CAD build for the part. Positions are in the model's coordinates, mm. Face numbers are marked on the shaded views. A direction names the side the tool comes from. Round coordinates to 2 decimals unless told otherwise and drop trailing zeros. Loops run counter-clockwise (first coordinate to the right, second up) from the corner with the lowest first, then second, coordinate; pieces in that order, holes last. Notation, with made-up numbers: M 40,61.25 L 89,61.25 A18 cw 89,94.25 Z; hole C 12,33 d8. An arc over 180 degrees is marked long. Use one line per item in the form item = value.
from build123d import *

# Parameters (mm, degrees)
F0_R     = 7.9375
F1_DEPTH = 3.175
F2_R     = 5.55625
F3_DEPTH = 11.1125
F5_DEPTH = 6.35
F6_SIZE  = 0.508


with BuildPart() as f1:
    # F0 (on Top) → F1 (new body)
    with BuildSketch(Plane.XY):
        Circle(F0_R)
    extrude(amount=F1_DEPTH)

    # F2 (on face) → F3 (join)
    with BuildSketch(Plane.XY.offset(3.175)):
        Circle(F2_R)
    extrude(amount=F3_DEPTH)

    # F4 (on face) → F5 (cut)
    with BuildSketch(Plane(origin=(0, 0, 0), x_dir=(1, 0, 0), z_dir=(0, 0, -1))):
        Polygon((-3.056609, -1.764734), (0, -3.529468), (3.056609, -1.764734), (3.056609, 1.764734), (0, 3.529468), (-3.056609, 1.764734), align=None)
    extrude(amount=-F5_DEPTH, mode=Mode.SUBTRACT)

    # F6
    f6_edges = [f1.edges().sort_by_distance(p)[0] for p in [
        (-5.55625, 0, 14.2875),
        (-7.9375, 0, 0),
    ]]
    chamfer(f6_edges, length=F6_SIZE)


solid = f1.part
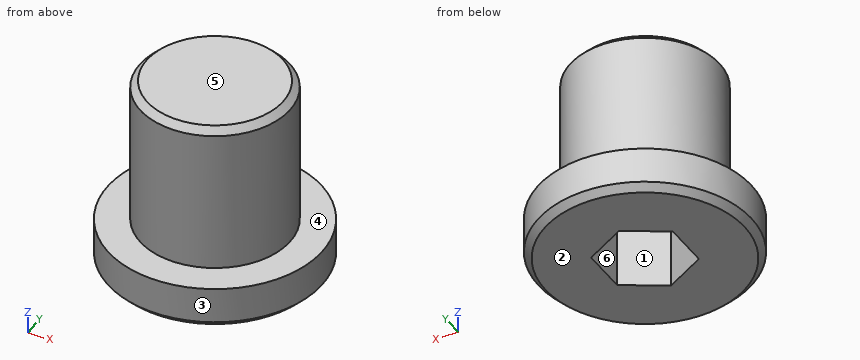
1. Probe line 1 along Z through (x, y) = (-3, -5.75) (3 decimals); line 2 along Y through (x, z) = (-1, 1.75); line 3 along X through (y, z) = (1.75, 9). List the from-to ranges inside material, lowest first. Write a range as from..to.
Completed:
line_1 = 0..3.175
line_2 = -7.87..-2.95, 2.95..7.87
line_3 = -5.27..5.27
2. Tool access for the marked faces 4, 5 and 6: list every direction of +Z, -Z, +X, -X, +Y, -Y with a clear straight run to the whole face (end or side of a thin tool).
Completed:
face_4 = +Z
face_5 = +Z, +X, -X, +Y, -Y
face_6 = -Z
3. Pull direction X, two halves, no side cores. Call the marked faces 1, 2 and 3: +X half, -X half, draft (parallel to the pull), parting line (faces both ways), or undercut.
Completed:
face_1 = undercut
face_2 = draft
face_3 = parting line
4. Cut at A-A on z = 4. Write the cut outline in (x, y), and give its area (3 significant figures).
Completed:
outline = C 0,0 d11.11; hole M -3.06,-1.76 L 0,-3.53 L 3.06,-1.76 L 3.06,1.76 L 0,3.53 L -3.06,1.76 Z
area = 64.6 mm2
5. Cut at C-C on z = 11.25. Write the cut outline in (x, y), and give its area (3 significant figures).
Completed:
outline = C 0,0 d11.11
area = 97.0 mm2
6. Drop flat-ended pins along their axis: P1, Ø1.5, axis at x = 6.5, y = 5, coming from the +Z side (3 decimals); P2, Ø6, axis at y = 5, z = 6.5, coming from the -X side; P3, Ø2, axis at x = 4, z = 12, coming from the +Y side. Give the stop position or say it passes through.
Completed:
P1 = 3.175
P2 = -5.18
P3 = 4.68
